Check sheet for the modelled part. Datum: model origin and axes. Units: mm. Face numbers are marked on the shaded views. Coordinates: 2 decimals unless noted, no trailing zeros. Loops run counter-clockwise (first coordinate to the right, second up) from the corner with the lowest first, then second, coordinate; pieces in that order, holes last. Notation, with made-up numbers: (15, 46.25) - (32, 46.25) arc R16 cw to (32, 72.25) - close; hole circle Ø8 at (-32, 27). An arc over 180 degrees is marked (long way). Use a Markdown table: item, result. Add a question column.
1) Draft check along Y on the marked faces 1, 2 and 3. Enter one of: pulls with the +Y half, pulls with the -Y half, needs draft (parallel to the pull), parting line crosses it, or undercut.
2) Thickness scan on line 1 (Z direction, x = -25.25, y = 0.25); line 2 (Y direction, x = -24.13, z = 44.5); line 3 (Y direction, x = -24, z = 48). Record the ranges inside material, lowest first.
3) Go/stop test with flat-tipped pins: P1, Ø2, axis at x = -7, z = 15.5, coming from the +Y side; P2, Ø3.5, axis at x = -24, y = 3, coming from the -Z side; P3, Ø3, axis at x = -24.13, y = 2.73, coming from the -Z side. Record where each tip stops, or that it passes through.
4) Sectioned sample at C-C, the plane x = -19.75. Enter the section's corners in (y, z).
5) Sectioned sample at B-B, the plane x = -16.75. Enter the section's corners in (y, z).
from build123d import *

# Parameters (mm, degrees)
BRIDA_BASE1_DEPTH     = 50.8
CORTAR_EXTRUIR1_START = 25.4
CORTAR_EXTRUIR1_DEPTH = 12.7
MATRIZL1_COUNT        = 2
MATRIZL1_PITCH        = 25.4


# Read off the part's stored shape, not the designer's step: Cortar-Extruir1
# Sheet-metal steps are written as plain solids
with BuildPart() as part:
    # Croquis1 → Brida base1 (new body)
    with BuildSketch(Plane.XY):
        with BuildLine():
            Line((0, 0), (-17.751111243, 0))
            ThreePointArc((-17.751111243, 0), (-17.77989007, 0.001256511), (-17.808449872, 0.00501648))
            Line((-17.808449872, 0.00501648), (-24.405666482, 1.168283766))
            ThreePointArc((-24.405666482, 1.168283766), (-25.014357108, 4.05002443), (-22.578895558, 2.393684921))
            Line((-22.578895558, 2.393684921), (-21.089835293, 2.069223014))
            ThreePointArc((-21.089835293, 2.069223014), (-25.863339932, 5.315648452), (-24.670306305, -0.33256325))
            Line((-24.670306305, -0.33256325), (-18.073089694, -1.495830536))
            ThreePointArc((-18.073089694, -1.495830536), (-17.912715421, -1.516944209), (-17.751111243, -1.524))
            Line((-17.751111243, -1.524), (0, -1.524))
            Line((0, -1.524), (0, 0))
        make_face()
    extrude(amount=BRIDA_BASE1_DEPTH)

    # Cortar-Extruir1 outline → Cortar-Extruir1 (cut)
    with BuildSketch(Plane.XY.offset(CORTAR_EXTRUIR1_START)):
        with BuildLine():
            Line((-24.670306305, -0.33256325), (-20.8915, -0.998868756))
            Line((-20.8915, -0.998868756), (-20.626860177, 0.50197826))
            Line((-20.626860177, 0.50197826), (-24.405666482, 1.168283766))
            ThreePointArc((-24.405666482, 1.168283766), (-25.014357108, 4.05002443), (-22.578895558, 2.393684921))
            Line((-22.578895558, 2.393684921), (-21.089835293, 2.069223014))
            ThreePointArc((-21.089835293, 2.069223014), (-25.863339932, 5.315648452), (-24.670306305, -0.33256325))
        make_face()
    cortar_extruir1 = extrude(amount=CORTAR_EXTRUIR1_DEPTH, mode=Mode.SUBTRACT)

    # MatrizL1: Cortar-Extruir1 ×2
    with Locations(*[(0, 0, -i * MATRIZL1_PITCH) for i in range(1, MATRIZL1_COUNT)]):
        add(cortar_extruir1, mode=Mode.SUBTRACT)


solid = part.part
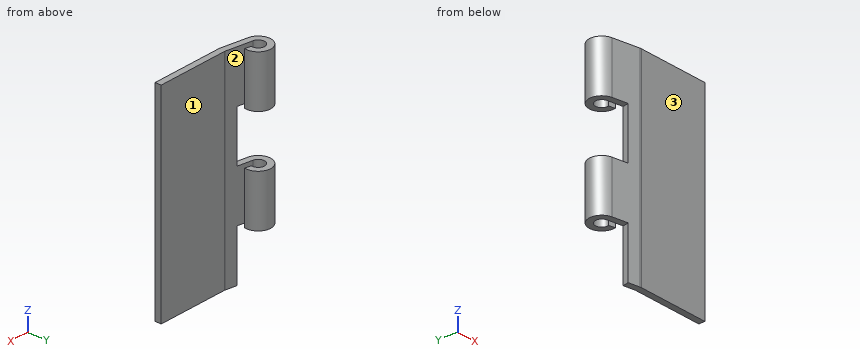
Solved:
| question | item | result |
|---|---|---|
| 1 | face 1 | pulls with the +Y half |
| 1 | face 2 | undercut |
| 1 | face 3 | pulls with the -Y half |
| 2 | line 1 | z = 12.7 to 25.4, 38.1 to 50.8 |
| 2 | line 2 | y = -0.43 to 1.12, 4.32 to 5.84 |
| 2 | line 3 | y = -0.45 to 1.1, 4.31 to 5.84 |
| 3 | P1 | stops at y = 0 |
| 3 | P2 | stops at z = 12.7 |
| 3 | P3 | passes through |
| 4 | outline | (-1.2, 0) - (0.35, 0) - (0.35, 50.8) - (-1.2, 50.8) - close |
| 5 | outline | (-1.52, 0) - (0, 0) - (0, 50.8) - (-1.52, 50.8) - close |
